Input: part model. Units: mm. Frame: model coordinates. Face numbers are marked on the shaded views. A direction names the side the tool comes from. Round coordinates to 2 decimals unless told otherwise and drop trailing zeros. Write each loop counter-clockwise with the first axis right and the second up, starting at its lowest first coordinate (ties: lowest second). Pieces come first, ordered by that corner, then holes. Notation, with made-up numbers: M 87.5,58 L 135.5,58 A20 ccw 135.5,77 Z; hole C 53.25,40 d3. An arc over 180 degrees is marked long. Write each question's results on one line, items separated by ' | '. Start each with the question number.
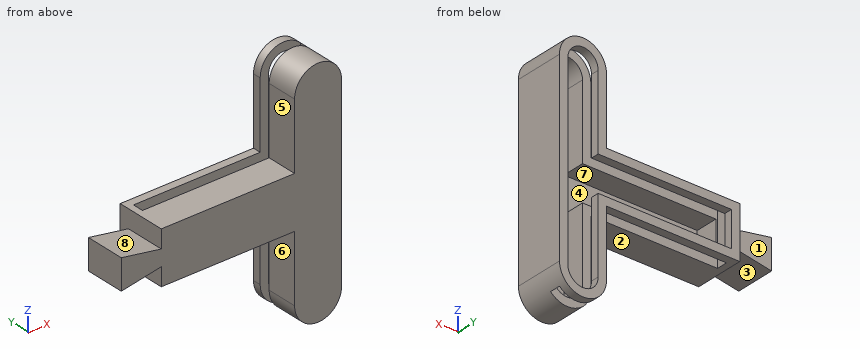
```python
from build123d import *

# Parameters (mm, degrees)
BOSS_EXTRUDE1_DEPTH      = 38.1
CUT_EXTRUDE10_DEPTH      = 7.62
SHELL2_START             = 6.35
SHELL2_DEPTH             = 31.75
SHELL2_2_DEPTH           = 17.78
CUT_EXTRUDE11_DEPTH      = 204.366887563
CUT_EXTRUDE11_DEPTH_BACK = 204.366887563
SKETCH6_W                = 127.254
SKETCH6_H                = 8.308241082


# Read off the part's stored shape, not the designer's step: Shell2
with BuildPart() as part:
    # Sketch1 → Boss-Extrude1 (new body)
    with BuildSketch(Plane(origin=(0, 0, 0), x_dir=(1, 0, 0), z_dir=(0, 1, 0))):
        with BuildLine():
            Line((0, 11.43), (0, -11.43))
            Line((0, -11.43), (30.48, -6.055553628))
            Line((30.48, -6.055553628), (30.48, -19.771553628))
            Line((30.48, -19.771553628), (132.08, -19.771553628))
            Line((132.08, -19.771553628), (132.08, -70.571553628))
            ThreePointArc((132.08, -70.571553628), (149.987, -88.478553628), (167.894, -70.571553628))
            Line((167.894, -70.571553628), (167.894, 70.571553628))
            ThreePointArc((167.894, 70.571553628), (149.987, 88.478553628), (132.08, 70.571553628))
            Line((132.08, 70.571553628), (132.08, 19.771553628))
            Line((132.08, 19.771553628), (30.48, 19.771553628))
            Line((30.48, 19.771553628), (30.48, 6.055553628))
            Line((30.48, 6.055553628), (0, 11.43))
        make_face()
    extrude(amount=BOSS_EXTRUDE1_DEPTH)

    # Sketch5 → Cut-Extrude10 (cut)
    with BuildSketch(Plane(origin=(0, 38.1, 0), x_dir=(1, 0, 0), z_dir=(0, 1, 0))):
        Polygon((0, -11.43), (0, 11.43), (0.205611809, 11.576348711), (30.48, 6.055553628), (30.48, -6.055553628), align=None)
    extrude(amount=-CUT_EXTRUDE10_DEPTH, mode=Mode.SUBTRACT)

    # Shell2 outline → Shell2 (cut)
    with BuildSketch(Plane(origin=(0, 0, 0), x_dir=(1, 0, 0), z_dir=(0, 1, 0)).offset(SHELL2_START)):
        with BuildLine():
            Line((36.83, 13.421553628), (36.83, -13.421553628))
            Line((36.83, -13.421553628), (138.43, -13.421553628))
            Line((138.43, -13.421553628), (138.43, -70.571553628))
            ThreePointArc((138.43, -70.571553628), (149.987, -82.128553628), (161.544, -70.571553628))
            Line((161.544, -70.571553628), (161.544, 70.571553628))
            ThreePointArc((161.544, 70.571553628), (149.987, 82.128553628), (138.43, 70.571553628))
            Line((138.43, 70.571553628), (138.43, 13.421553628))
            Line((138.43, 13.421553628), (36.83, 13.421553628))
        make_face()
    extrude(amount=SHELL2_DEPTH, mode=Mode.SUBTRACT)

    # Shell2 2 outline → Shell2 2 (cut)
    with BuildSketch(Plane(origin=(0, 0, 0), x_dir=(1, 0, 0), z_dir=(0, 1, 0)).offset(SHELL2_START)):
        Polygon((28.25455863, 0), (6.35, 3.862364687), (6.35, -3.862364687), align=None)
    extrude(amount=SHELL2_2_DEPTH, mode=Mode.SUBTRACT)

    # Sketch6 → Cut-Extrude11 (cut, two sides: drawn at the far end of the back side and taken through both)
    with BuildSketch(Plane.XY.offset(19.771553628).offset(-CUT_EXTRUDE11_DEPTH_BACK)):
        with Locations((99.187, 27.763521135)):
            Rectangle(SKETCH6_W, SKETCH6_H)
    extrude(amount=CUT_EXTRUDE11_DEPTH + CUT_EXTRUDE11_DEPTH_BACK, mode=Mode.SUBTRACT)


solid = part.part
```
1. Cut plane A-A on x = 130. Output: boundary loops of the cut face in (y, z), and give its area (3 significant figures).
2. Line query: L1, parallel to Z at x = 150.5, y = 23.5; L2, parallel to X at y = 31, z = -6; L3, parallel to X at y = 16, z = -13. Output: solid intervals per line, ascending. Write a range as from..to.
3. Cut plane C-C on y = 10. Output: boundary loops of the cut face in (x, z), and give its area (3 significant figures).
4. Draft query along Z for the marked faces 6, 7 and 8. Return one class per face: +Z half, -Z half, draft (parallel to the pull), parting line (faces both ways), or undercut.
5. Contact query for flat-ended pins moving along their axis: P1, Ø14, axis at x = 75.5, y = 15.5, coming from the +Z side; P2, Ø3, axis at x = 58.5, y = 29.5, coming from the -Z side; P3, Ø12, axis at x = 45.5, y = 26, coming from the -Z side; P4, Ø6, axis at x = 15.5, z = 0.5, coming from the +Y side. Output: stop coordinate, or through.
6. Cut plane D-D on x = 33. Output: boundary loops of the cut face in (y, z), and give its area (3 significant figures).
7. Access query for the marked faces 1, 2, 3, 4 and 5. Directions: +Z, -Z, +X, -X, +Y, -Y. A direction counts if a zero-diameter tool reaches every point of the face in a straight line with its end or side. Return the directions, or none.
8. Cut plane B-B on z = 30.5. Output: boundary loops of the cut face in (x, y).
Answers follow:
1) outline: M 0,-19.77 L 23.61,-19.77 L 23.61,-13.42 L 6.35,-13.42 L 6.35,13.42 L 23.61,13.42 L 23.61,19.77 L 0,19.77 Z; M 31.92,-19.77 L 38.1,-19.77 L 38.1,-13.42 L 31.92,-13.42 Z; M 31.92,13.42 L 38.1,13.42 L 38.1,19.77 L 31.92,19.77 Z | area: 549 mm2
2) L1: z = -88.47..-82.12, 82.12..88.47 | L2: x = 30.48..35.56, 162.81..167.89 | L3: x = 30.48..36.83, 161.54..167.89
3) outline: M 0,-11.43 L 30.48,-6.06 L 30.48,-19.77 L 132.08,-19.77 L 132.08,-70.57 A17.91 ccw 167.89,-70.57 L 167.89,70.57 A17.91 ccw 132.08,70.57 L 132.08,19.77 L 30.48,19.77 L 30.48,6.06 L 0,11.43 Z; hole M 6.35,-3.86 L 28.25,0 L 6.35,3.86 Z; hole M 36.83,-13.42 L 138.43,-13.42 L 138.43,-70.57 A11.56 ccw 161.54,-70.57 L 161.54,70.57 A11.56 ccw 138.43,70.57 L 138.43,13.42 L 36.83,13.42 Z | area: 4,120 mm2
4) face 6: draft | face 7: undercut | face 8: +Z half
5) P1: stops at z = 19.77 | P2: passes through | P3: stops at z = -19.77 | P4: stops at y = 30.48
6) outline: M 0,-19.77 L 38.1,-19.77 L 38.1,19.77 L 0,19.77 Z | area: 1,510 mm2
7) face 1: +Z, -Z, -X, +Y | face 2: -Z, -X, +Y, -Y | face 3: -Z, +Y, -Y | face 4: +Y | face 5: +Z, -X, +Y, -Y
8) outline: M 132.08,0 L 167.89,0 L 167.89,38.1 L 161.54,38.1 L 161.54,31.92 L 162.81,31.92 L 162.81,23.61 L 161.54,23.61 L 161.54,6.35 L 138.43,6.35 L 138.43,23.61 L 132.08,23.61 Z; M 132.08,31.92 L 138.43,31.92 L 138.43,38.1 L 132.08,38.1 Z
